Work out the finished part from the listing and answer in its coordinate system (mm). Coordinates: 2 decimals unless noted, no trailing zeros. Write each loop counter-clockwise with the first axis right and the second up, starting at its lowest first coordinate (ties: lowest second). Pieces come first, ordered by that corner, then holes. Notation, with made-up numbers: (58.25, -35.5) - (108.25, -35.5) arc R27 ccw to (108.25, -14.5) - close; hole circle Ø8 at (-24, 50). An arc over 180 degrees is marked (long way). Use a Markdown table: item, result. Add a question column.
(1) Find the intervals of material crossed by line 1 (Y direction, x = 33, z = -34.5); line 2 (X direction, y = -3, z = -34); line 3 (X direction, y = -2.65, z = -14), in increasing order. Write a range as from..to.
(2) The part is cut by section A-A, the plane x = 11.5. Give the vertices of the cut face in (y, z).
(3) The part is cut by section C-C, the plane y = -2.3. Give the vertices of the cut face in (x, z), then the cut area to 3 significant figures.
(4) Given pin 1 Ø10 at (x, z) = (30.5, -36) entering from +Y; pin 2 Ø1.5 at (y, z) = (-3, -39.5) entering from +X, each flat-ended and moving along its own axis, determine where each tip first touches the part or whether it passes through.
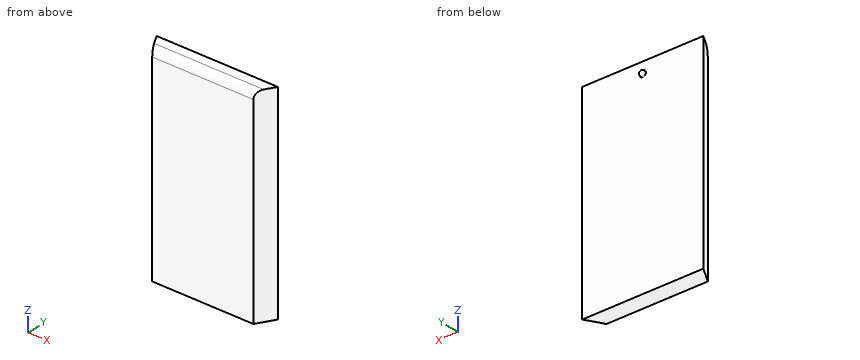
Autodesk Inventor part; units mm, degrees
ref_plane "Work Plane1" through (22.2652, -0.25, -3) normal (0, 0, 1) x (1, 0, 0)
ref_plane "YZ Plane" through (0, 0, 0) normal (1, 0, 0) x (0, 1, 0)
ref_plane "XZ Plane" through (0, 0, 0) normal (0, 1, 0) x (-1, 0, 0)
sketch "Sketch1" plane through (0, 0, 0) normal (0, 0, 1) x (1, 0, 0)
  line L0 (39.4171, 0) -> (37.6851, -3)
  line L1 (6.8453, -3) -> (5.1132, 0)
  line L2 (5.1132, 0) -> (39.4171, 0)
  line L3 (36.3139, -4.875) -> (38.9841, -0.25)
  line L4 (38.9841, -0.25) -> (5.5463, -0.25)
  line L5 (5.5463, -0.25) -> (8.2165, -4.875)
  line L6 (36.3139, -4.875) -> (36.2417, -5)
  line L7 (8.2165, -4.875) -> (8.2887, -5)
  line L8 (8.2887, -5) -> (36.2417, -5)
  point P0 (0, 0)
  dimension "d0" = 0.25
  dimension "d1" = 4.75
extrude "Extrusion1" add sketch "Sketch1" against normal blind 57
sketch "Sketch2" plane through (5.5463, -0.25, 0) normal (0, 1, 0) x (1, 0, 0)
  circle A0 centre (16.7189, 3) radius 0.922
  point P0 (-5.5463, 0)
ref_plane "Work Plane1" through (22.2652, -0.25, -3) normal (0, 0, 1) x (1, 0, 0)
sketch "Sketch3" plane through (22.2652, -0.25, -3) normal (0, 0, 1) x (1, 0, 0)
  line L0 (-16.7189, 0) -> (16.7189, 0) construction
  line L1 (0, 0) -> (0, 0.85) construction
  arc A0 (0.7775, 0.3597) -> (-0.7775, 0.3597) centre (0, 0.1429) ccw construction
  arc A1 (0, 0.85) -> (-0.75, 0) centre (0, 0.0941) ccw
  line L2 (-0.75, 0) -> (0, 0)
  line L3 (0, 0) -> (0, 0.85)
  point P0 (-22.2652, 0.25)
  dimension "d4" = 0.85
  dimension "d5" = 0.75
revolve "Revolution1" add sketch "Sketch3" angle 360 about axis through (22.2652, -0.25, -3) along (0, 1, 0)
fillet "Fillet1" radius 0.18 1 edges at (23.0152, -0.25, -3)
fillet "Fillet2" radius 2 1 edges at (22.2652, -5, 0)
Model answer:
| question | item | result |
|---|---|---|
| 1 | line 1 | -5..-0.25 |
| 1 | line 2 | 7.13..37.4 |
| 1 | line 3 | 6.93..37.6 |
| 2 | outline | (-5, -57) - (-0.25, -57) - (-0.25, 0) - (-3, 0) arc R2 ccw to (-5, -2) - close |
| 3 | outline | (6.73, -57) - (37.8, -57) - (37.8, 0) - (6.73, 0) - close |
| 3 | area | 1,770 mm^2 |
| 4 | pin 1 | y = -0.25 |
| 4 | pin 2 | x = 37.83 |
